```python
from build123d import *

# Parameters (mm, degrees)
F0_R       = 5
F1_DEPTH   = 3.75
F0_W       = 3.02
F0_H       = 16.12
F2_DEPTH   = 25.93
F3_DEPTH   = 6.79
F4_DEPTH   = 6.79
F5_SIZE2   = 3.03999
F5_SIZE    = 2.64999
F5_2_SIZE2 = 3.03999
F5_2_SIZE  = 2.64999
F6_SIZE2   = 2.64999
F6_SIZE    = 3.03999
F6_2_SIZE2 = 2.64999
F6_2_SIZE  = 3.03999
F7_R       = 2.33
F8_DEPTH   = 25
F9_R       = 8.05999
F10_R      = 5
F11_R      = 10.89999


# Not quite as in the source:
# - a fillet or chamfer is up to 0.001 mm smaller than in the source, because OpenCascade refuses the exact size


with BuildPart() as f1:
    # F0 (on Top) → F1 (new body)
    with BuildSketch(Plane.XY):
        Polygon((-30.935, 0), (-12.725, 0), (12.725, 0), (30.935, 0), (30.935, 21.8), (-30.935, 21.8), align=None)
        with BuildLine():
            ThreePointArc((-11.9316907323, 12.91), (-11.7843146524, 12.0027843216), (-11.735, 11.085))
            ThreePointArc((-11.735, 11.085), (-11.8230688054, 9.8599030561), (-12.0854641032, 8.66))
            ThreePointArc((-12.0854641032, 8.66), (-12.4738263465, 7.6050242897), (-12.9970143092, 6.61))
            ThreePointArc((-12.9970143092, 6.61), (-20.3, 2.52), (-27.6029856908, 6.61))
            ThreePointArc((-27.6029856908, 6.61), (-28.1261736535, 7.6050242897), (-28.5145358968, 8.66))
            ThreePointArc((-28.5145358968, 8.66), (-28.8593991283, 10.7753040808), (-28.6683092677, 12.91))
            ThreePointArc((-28.6683092677, 12.91), (-28.2468859573, 14.2797188579), (-27.6029856908, 15.56))
            ThreePointArc((-27.6029856908, 15.56), (-20.3, 19.65), (-12.9970143092, 15.56))
            ThreePointArc((-12.9970143092, 15.56), (-12.3531140427, 14.2797188579), (-11.9316907323, 12.91))
        make_face(mode=Mode.SUBTRACT)
        with BuildLine():
            ThreePointArc((28.6065440218, 12.91), (28.8001487986, 11.8553299132), (28.865, 10.785))
            ThreePointArc((28.865, 10.785), (28.8001487986, 9.7146700868), (28.6065440218, 8.66))
            ThreePointArc((28.6065440218, 8.66), (28.2771488358, 7.6105658536), (27.8203324738, 6.61))
            ThreePointArc((27.8203324738, 6.61), (20, 1.92), (12.1796675262, 6.61))
            ThreePointArc((12.1796675262, 6.61), (11.7228511642, 7.6105658536), (11.3934559782, 8.66))
            ThreePointArc((11.3934559782, 8.66), (11.135, 10.785), (11.3934559782, 12.91))
            ThreePointArc((11.3934559782, 12.91), (11.8536949602, 14.2815610531), (12.5308902806, 15.56))
            ThreePointArc((12.5308902806, 15.56), (20, 19.65), (27.4691097194, 15.56))
            ThreePointArc((27.4691097194, 15.56), (28.1463050398, 14.2815610531), (28.6065440218, 12.91))
        make_face(mode=Mode.SUBTRACT)
        Polygon((12.725, 0), (-12.725, 0), (-12.725, -10.84), (-9.705, -10.84), (-9.705, -26.96), (-12.725, -26.96), (-12.725, -63.35), (12.725, -63.35), (12.725, -26.96), (9.705, -26.96), (9.705, -10.84), (12.725, -10.84), align=None)
        with Locations((0, -35.12)):
            Circle(F0_R, mode=Mode.SUBTRACT)
        with BuildLine():
            ThreePointArc((-12.0854641032, 8.66), (-11.8230688054, 9.8599030561), (-11.735, 11.085))
            ThreePointArc((-11.735, 11.085), (-11.7843146524, 12.0027843216), (-11.9316907323, 12.91))
            Line((-11.9316907323, 12.91), (-28.6683092677, 12.91))
            ThreePointArc((-28.6683092677, 12.91), (-28.8593991283, 10.7753040808), (-28.5145358968, 8.66))
            Line((-28.5145358968, 8.66), (-12.0854641032, 8.66))
        make_face()
        with BuildLine():
            ThreePointArc((28.6065440218, 8.66), (28.8001487986, 9.7146700868), (28.865, 10.785))
            ThreePointArc((28.865, 10.785), (28.8001487986, 11.8553299132), (28.6065440218, 12.91))
            Line((28.6065440218, 12.91), (11.3934559782, 12.91))
            ThreePointArc((11.3934559782, 12.91), (11.135, 10.785), (11.3934559782, 8.66))
            Line((11.3934559782, 8.66), (28.6065440218, 8.66))
        make_face()
    extrude(amount=F1_DEPTH)

    # F0 (on Top) → F2 (join)
    with BuildSketch(Plane.XY):
        with Locations((-11.215, -18.9)):
            Rectangle(F0_W, F0_H)
        with Locations((11.215, -18.9)):
            Rectangle(F0_W, F0_H)
    extrude(amount=F2_DEPTH)

    # F0 (on Top) → F3 (join)
    with BuildSketch(Plane.XY):
        with BuildLine():
            Line((-27.6029856908, 15.56), (-12.9970143092, 15.56))
            ThreePointArc((-12.9970143092, 15.56), (-20.3, 19.65), (-27.6029856908, 15.56))
        make_face()
        with BuildLine():
            ThreePointArc((-27.6029856908, 6.61), (-20.3, 2.52), (-12.9970143092, 6.61))
            Line((-12.9970143092, 6.61), (-27.6029856908, 6.61))
        make_face()
        with BuildLine():
            ThreePointArc((12.1796675262, 6.61), (20, 1.92), (27.8203324738, 6.61))
            Line((27.8203324738, 6.61), (12.1796675262, 6.61))
        make_face()
        with BuildLine():
            Line((12.5308902806, 15.56), (27.4691097194, 15.56))
            ThreePointArc((27.4691097194, 15.56), (20, 19.65), (12.5308902806, 15.56))
        make_face()
    extrude(amount=F3_DEPTH)

    # F0 (on Top) → F4 (join)
    with BuildSketch(Plane.XY):
        with BuildLine():
            Line((-28.6683092677, 12.91), (-11.9316907323, 12.91))
            ThreePointArc((-11.9316907323, 12.91), (-12.3531140427, 14.2797188579), (-12.9970143092, 15.56))
            Line((-12.9970143092, 15.56), (-27.6029856908, 15.56))
            ThreePointArc((-27.6029856908, 15.56), (-28.2468859573, 14.2797188579), (-28.6683092677, 12.91))
        make_face()
        with BuildLine():
            ThreePointArc((-12.9970143092, 6.61), (-12.4738263465, 7.6050242897), (-12.0854641032, 8.66))
            Line((-12.0854641032, 8.66), (-28.5145358968, 8.66))
            ThreePointArc((-28.5145358968, 8.66), (-28.1261736535, 7.6050242897), (-27.6029856908, 6.61))
            Line((-27.6029856908, 6.61), (-12.9970143092, 6.61))
        make_face()
        with BuildLine():
            ThreePointArc((27.8203324738, 6.61), (28.2771488358, 7.6105658536), (28.6065440218, 8.66))
            Line((28.6065440218, 8.66), (11.3934559782, 8.66))
            ThreePointArc((11.3934559782, 8.66), (11.7228511642, 7.6105658536), (12.1796675262, 6.61))
            Line((12.1796675262, 6.61), (27.8203324738, 6.61))
        make_face()
        with BuildLine():
            Line((11.3934559782, 12.91), (28.6065440218, 12.91))
            ThreePointArc((28.6065440218, 12.91), (28.1463050398, 14.2815610531), (27.4691097194, 15.56))
            Line((27.4691097194, 15.56), (12.5308902806, 15.56))
            ThreePointArc((12.5308902806, 15.56), (11.8536949602, 14.2815610531), (11.3934559782, 12.91))
        make_face()
    extrude(amount=F4_DEPTH)

    # F5 (size 2.65 and 3.04 in the source; OpenCascade refuses exactly that, so slightly less here)
    f5_edges = [f1.edges().sort_by_distance(p)[0] for p in [
        (-20.3, 12.91, 6.79),
    ]]
    f5_side = f1.faces().sort_by_distance((-20.3, 15.724453, 6.79))[0]
    chamfer(f5_edges, length=F5_SIZE, length2=F5_SIZE2, reference=f5_side)

    # F5#2 (size 2.65 and 3.04 in the source; OpenCascade refuses exactly that, so slightly less here)
    f5_2_edges = [f1.edges().sort_by_distance(p)[0] for p in [
        (20, 12.91, 6.79),
    ]]
    f5_2_side = f1.faces().sort_by_distance((20, 15.719253, 6.79))[0]
    chamfer(f5_2_edges, length=F5_2_SIZE, length2=F5_2_SIZE2, reference=f5_2_side)

    # F6 (size 3.04 and 2.65 in the source; OpenCascade refuses exactly that, so slightly less here)
    f6_edges = [f1.edges().sort_by_distance(p)[0] for p in [
        (-20.3, 8.66, 6.79),
    ]]
    f6_side = f1.faces().sort_by_distance((-20.3, 8.66, 5.27))[0]
    chamfer(f6_edges, length=F6_SIZE, length2=F6_SIZE2, reference=f6_side)

    # F6#2 (size 3.04 and 2.65 in the source; OpenCascade refuses exactly that, so slightly less here)
    f6_2_edges = [f1.edges().sort_by_distance(p)[0] for p in [
        (20, 8.66, 6.79),
    ]]
    f6_2_side = f1.faces().sort_by_distance((20, 8.66, 5.27))[0]
    chamfer(f6_2_edges, length=F6_2_SIZE, length2=F6_2_SIZE2, reference=f6_2_side)

    # F7 (on face) → F8 (cut)
    with BuildSketch(Plane(origin=(-12.725, 0, 0), x_dir=(0, -1, 0), z_dir=(-1, 0, 0))):
        with Locations((18.9, 17.99)):
            Circle(F7_R)
    extrude(amount=-F8_DEPTH, mode=Mode.SUBTRACT)

    # F9 (radius 8.06 in the source; OpenCascade refuses exactly that, so slightly less here)
    f9_edges = [f1.edges().sort_by_distance(p)[0] for p in [
        (-11.215, -10.84, 25.93),
        (11.215, -10.84, 25.93),
        (11.215, -26.96, 25.93),
        (-11.215, -26.96, 25.93),
    ]]
    fillet(f9_edges, radius=F9_R)

    # F10
    f10_edges = [f1.edges().sort_by_distance(p)[0] for p in [
        (-12.725, 0, 1.875),
        (12.725, 0, 1.875),
        (12.725, -63.35, 1.875),
        (-12.725, -63.35, 1.875),
        (-11.215, -26.96, 3.75),
        (11.215, -26.96, 3.75),
        (11.215, -10.84, 3.75),
        (-11.215, -10.84, 3.75),
    ]]
    fillet(f10_edges, radius=F10_R)

    # F11 (radius 10.9 in the source; OpenCascade refuses exactly that, so slightly less here)
    f11_edges = [f1.edges().sort_by_distance(p)[0] for p in [
        (-30.935, 21.8, 1.875),
        (-30.935, 0, 1.875),
        (30.935, 21.8, 1.875),
        (30.935, 0, 1.875),
    ]]
    fillet(f11_edges, radius=F11_R)


solid = f1.part
```
Geometry: final body of the model. Coordinates: model frame, mm. A direction names the side the tool comes from. Round coordinates to 2 decimals unless told otherwise and drop trailing zeros. Loops run counter-clockwise (first coordinate to the right, second up) from the corner with the lowest first, then second, coordinate; pieces in that order, holes last.
Item 1: Contact query for flat-ended pins moving along their axis: P1, Ø5, axis at y = -35, z = 6, coming from the -X side (3 decimals); P2, Ø2.5, axis at x = -19, z = 1.5, coming from the -Y side; P3, Ø1.4, axis at y = -19, z = 18, coming from the -X side (3 decimals). Output: stop coordinate, or through.
Checked values:
P1: stops at x = -12.725
P2: stops at y = 0
P3: stops at x = 12.275
Item 2: Section B-B, the plane y = -35.12. Output: boundary loops of the cut face in (x, z) (3 decimals), plus the area to 3 significant figures.
Checked values:
outline: (-12.725, 0) - (-5, 0) - (-5, 3.75) - (-12.725, 3.75) - close; (5, 0) - (12.725, 0) - (12.725, 3.75) - (5, 3.75) - close
area: 57.9 mm2
Item 3: Line query: L1, parallel to X at y = -14, z = 23.5 (3 decimals); L2, parallel to Y at x = 0, z = 2.25; L3, parallel to Z at x = -1.5, y = 18.5. Output: solid intervals per line, ascending.
Checked values:
L1: x = -12.725 to -9.705, 9.705 to 12.725
L2: y = -63.35 to -40.12, -30.12 to 21.8
L3: z = 0 to 3.75
Item 4: Section A-A, the plane x = 0. Output: boundary loops of the cut face in (y, z).
Checked values:
outline: (-63.35, 0) - (-40.12, 0) - (-40.12, 3.75) - (-63.35, 3.75) - close; (-30.12, 0) - (21.8, 0) - (21.8, 3.75) - (-30.12, 3.75) - close
Item 5: Mould query, pull axis X, two halves, no side actions, for faces 1 (the flat face through (0, -11, 3.75)), 2 (the cylindrical face through (11.221, -61.924, 1.901)), 3 (the cylindrical face through (11.24, -24.66, 23.51)). Classes: released by +X, released by -X, zero draft, split by the parting line, or undercut.
Checked values:
face 1: undercut
face 2: released by +X
face 3: zero draft
Item 6: Reachability of faces 4 (the flat face through (11, -10.84, 13)), 5 (the flat face through (-11, -26.96, 13)), 6 (the flat face through (-20, 14, 5)), 7 (the flat face through (9.705, -19, 15)) from +Z, -Z, +X, -X, +Y, -Y: full face, straight path, thin tool, end or side. Return the list, or none.
Checked values:
face 4: +Z, +X, -X, +Y
face 5: +Z, +X, -X, -Y
face 6: +Z, +X, -X
face 7: +Z, +Y, -Y
